```python
from build123d import *

# Parameters (mm, degrees)
F0_R         = 3.5
F0_R_2       = 2.8
F1_DEPTH     = 12
F3_DEPTH     = 1.7
F5_DEPTH     = 0.7
F6_T4_DEPTH  = 6.526963201
F6_S5_R      = 2.8
F6_T6_DEPTH  = 5
F6_T10_DEPTH = 6.526963201
F6_S11_R     = 2.8
F6_T12_DEPTH = 5
F6_T16_DEPTH = 6.526963201
F6_S17_R     = 2.8
F6_T18_DEPTH = 5
F6_T22_DEPTH = 6.526963201
F6_S23_R     = 2.8
F6_T24_DEPTH = 5
F7_T2_ANGLE  = 236.1398810925
F7_T4_ANGLE  = 236.1398810925


# Not quite as in the source:
# - a fillet or chamfer that OpenCascade refuses, or shapes differently, is made with other operations: its cross-section is extruded or revolved along the edge and cut away or added
# - a pattern or mirror of a feature is missing from the dataset's text; its kind, count and spacing are read off the source's solid


with BuildPart() as f1:
    # F0 (on Top) → F1 (new body)
    with BuildSketch(Plane.XY):
        Polygon((3.1971086236, -5.9505038819), (6.7518418389, -0.2064746542), (3.5547332152, 5.7440292277), (-3.1971086236, 5.9505038819), (-6.7518418389, 0.2064746542), (-3.5547332152, -5.7440292277), align=None)
        Circle(F0_R, mode=Mode.SUBTRACT)
        Circle(F0_R)
        Circle(F0_R_2, mode=Mode.SUBTRACT)
    extrude(amount=F1_DEPTH)

    # F2 (on face) → F3 (cut)
    with BuildSketch(Plane(origin=(0, 0, 0), x_dir=(1, 0, 0), z_dir=(0, 0, -1))):
        with BuildLine():
            Line((-5.3518418389, -1.1), (-2.5748786379, -1.1))
            ThreePointArc((-2.5748786379, -1.1), (-2.8, 0), (-2.5748786379, 1.1))
            Line((-2.5748786379, 1.1), (-5.3518418389, 1.1))
            Line((-5.3518418389, 1.1), (-5.3518418389, -1.1))
        make_face()
        with BuildLine():
            Line((2.5748786379, -1.1), (5.3518418389, -1.1))
            Line((5.3518418389, -1.1), (5.3518418389, 1.1))
            Line((5.3518418389, 1.1), (2.5748786379, 1.1))
            ThreePointArc((2.5748786379, 1.1), (2.7431423756, 0.5613999527), (2.8, 0))
            ThreePointArc((2.8, 0), (2.7431423756, -0.5613999527), (2.5748786379, -1.1))
        make_face()
    extrude(amount=-F3_DEPTH, mode=Mode.SUBTRACT)

    # F4 (on face) → F5 (join)
    with BuildSketch(Plane(origin=(0, 0, 0), x_dir=(1, 0, 0), z_dir=(0, 0, -1))):
        with BuildLine():
            ThreePointArc((-3.6402666737, -1.1), (0, -3.8028333457), (3.6402666737, -1.1))
            Line((3.6402666737, -1.1), (2.5748786379, -1.1))
            ThreePointArc((2.5748786379, -1.1), (0, -2.8), (-2.5748786379, -1.1))
            Line((-2.5748786379, -1.1), (-3.6402666737, -1.1))
        make_face()
    f5 = extrude(amount=F5_DEPTH)

    # F5_copies: F5 across plane
    add(f5.mirror(Plane(origin=(0, 0, 0), x_dir=(0, 0, -1), z_dir=(0, -1, 0))))

    # F6: fillet of radius 1.5 on 4 edges, made by hand


with BuildPart() as f6_tool2:
    # F6_s3 → F6_t4 (new body)
    with BuildSketch(Plane.YZ.offset(-1.1751213621)):
        with BuildLine():
            ThreePointArc((1.1, 0.2), (0.6606601718, 1.2606601718), (-0.4, 1.7))
            Line((-0.4, 1.7), (1.1, 1.7))
            Line((1.1, 1.7), (1.1, 0.2))
        make_face()
    extrude(amount=F6_T4_DEPTH)

    # F6_s5 → F6_t6 (cut, symmetric)
    with BuildSketch(Plane.XY.offset(1)):
        Circle(F6_S5_R)
    extrude(amount=F6_T6_DEPTH, both=True, mode=Mode.SUBTRACT)


with BuildPart() as f1_1:
    add(f1.part)

    # F6_t1: union F6_tool2
    add(f6_tool2.part)


with BuildPart() as f6_tool8:
    # F6_s9 → F6_t10 (new body)
    with BuildSketch(Plane.YZ.offset(-5.3518418389)):
        with BuildLine():
            ThreePointArc((1.1, 0.2), (0.6606601718, 1.2606601718), (-0.4, 1.7))
            Line((-0.4, 1.7), (1.1, 1.7))
            Line((1.1, 1.7), (1.1, 0.2))
        make_face()
    extrude(amount=F6_T10_DEPTH)

    # F6_s11 → F6_t12 (cut, symmetric)
    with BuildSketch(Plane.XY.offset(1)):
        Circle(F6_S11_R)
    extrude(amount=F6_T12_DEPTH, both=True, mode=Mode.SUBTRACT)


with BuildPart() as f1_2:
    add(f1_1.part)

    # F6_t7: union F6_tool8
    add(f6_tool8.part)


with BuildPart() as f6_tool14:
    # F6_s15 → F6_t16 (new body)
    with BuildSketch(Plane.YZ.offset(5.3518418389)):
        with BuildLine():
            ThreePointArc((-1.1, 0.2), (-0.6606601718, 1.2606601718), (0.4, 1.7))
            Line((0.4, 1.7), (-1.1, 1.7))
            Line((-1.1, 1.7), (-1.1, 0.2))
        make_face()
    extrude(amount=-F6_T16_DEPTH)

    # F6_s17 → F6_t18 (cut, symmetric)
    with BuildSketch(Plane.XY.offset(1)):
        Circle(F6_S17_R)
    extrude(amount=F6_T18_DEPTH, both=True, mode=Mode.SUBTRACT)


with BuildPart() as f1_3:
    add(f1_2.part)

    # F6_t13: union F6_tool14
    add(f6_tool14.part)


with BuildPart() as f6_tool20:
    # F6_s21 → F6_t22 (new body)
    with BuildSketch(Plane.YZ.offset(1.1751213621)):
        with BuildLine():
            ThreePointArc((-1.1, 0.2), (-0.6606601718, 1.2606601718), (0.4, 1.7))
            Line((0.4, 1.7), (-1.1, 1.7))
            Line((-1.1, 1.7), (-1.1, 0.2))
        make_face()
    extrude(amount=-F6_T22_DEPTH)

    # F6_s23 → F6_t24 (cut, symmetric)
    with BuildSketch(Plane.XY.offset(1)):
        Circle(F6_S23_R)
    extrude(amount=F6_T24_DEPTH, both=True, mode=Mode.SUBTRACT)


with BuildPart() as f1_4:
    add(f1_3.part)

    # F6_t19: union F6_tool20
    add(f6_tool20.part)

    # F7: fillet of radius 1 on 2 edges, made by hand

    # F7_s1 → F7_t2 (revolve, cut)
    with BuildSketch(Plane(origin=(0, 0, 0), x_dir=(0, 0, 1), z_dir=(-0.4705490205, -0.8823738546, 0))):
        with BuildLine():
            ThreePointArc((0.3, -2.8), (-0.4071067812, -3.0928932188), (-0.7, -3.8))
            Line((-0.7, -3.8), (-0.7, -2.8))
            Line((-0.7, -2.8), (0.3, -2.8))
        make_face()
    revolve(axis=Axis((0, 0, -0.7), (0, 0, 1)), revolution_arc=F7_T2_ANGLE, mode=Mode.SUBTRACT)

    # F7_s3 → F7_t4 (revolve, cut)
    with BuildSketch(Plane(origin=(0, 0, 0), x_dir=(0, 0, 1), z_dir=(-0.4705490205, 0.8823738546, 0))):
        with BuildLine():
            ThreePointArc((0.3, 2.8), (-0.4071067812, 3.0928932188), (-0.7, 3.8))
            Line((-0.7, 3.8), (-0.7, 2.8))
            Line((-0.7, 2.8), (0.3, 2.8))
        make_face()
    revolve(axis=Axis((0, 0, -0.7), (0, 0, -1)), revolution_arc=F7_T4_ANGLE, mode=Mode.SUBTRACT)


solid = f1_4.part
```
Could you check a few things on this model? Use its own coordinates, in mm. A direction names the side the tool comes from. Coordinates: 2 decimals unless noted, no trailing zeros. Write each loop counter-clockwise with the first axis right and the second up, starting at its lowest first coordinate (ties: lowest second). Pieces come first, ordered by that corner, then holes. Notation, with made-up numbers: M -24,55.5 L -4,55.5 A20 ccw -4,68.5 Z; hole C 16,-20 d10. An arc over 180 degrees is marked long. Answer as CSV lines item,"result". Start each with the question number.
1) Please list where these lines run through material, in increasing order: line 1 (Z direction, x = 3, y = 3.25); line 2 (Y direction, x = 2.5, z = 9.25); line 3 (Y direction, x = 0, z = 7). Write a range as from..to.
2) We'd pull the mould along X, two halves only. Please class faces 1 (the flat face through (3, -1.1, 0)), 2 (the flat face through (3, 0, 12)), 3 (the flat face through (-4.95, 3.12, 5.92)): +X half, -X half, draft (parallel to the pull), parting line (faces both ways), or undercut.
3) I want a section at D-D, the plane z = 1. Please give me the cut outline in (x, y), and give its area (3 significant figures).
4) For faces 4 (the cylindrical face through (-0.1, -3.8, -0.3)), 5 (the flat face through (5.176, 2.727, 5.916)), 6 (the flat face through (-5.176, -2.727, 5.916)), 7 (the cylindrical face through (-0.1, 3.8, -0.3)), 8 (the cylindrical face through (4, -0.8, 1.1)), which set-ups out of +Z, -Z, +X, -X, +Y, -Y let a thin tool reach every point of the face, with its end or its side?
5) I want a section at A-A, the plane z = 11. Please give me the cut outline in (x, y), and give its area (3 significant figures).
6) For P1, Ø0.5, axis at x = -4, z = 0, coming from the -Y side; P2, Ø2, axis at y = -4, z = 9.5, coming from the -X side; P3, Ø0.8, axis at y = -0.5, z = 1, coming from the -X side; P4, Ø5, axis at x = 4, z = 5, coming from the -Y side, each with a flat end and sliding along its axis, tell me the tip position at first contact or that it passes through.
7) I want a section at C-C, the plane x = -4.25. Please give me the cut outline in (y, z), and give its area (3 significant figures).
Data:
1,line 1,"z = 0..12"
1,line 2,"y = -5.93..-1.26, 1.26..5.78"
1,line 3,"y = -5.85..-2.8, 2.8..5.85"
2,face 1,"undercut"
2,face 2,"draft"
2,face 3,"-X half"
3,outline,"M -6.75,0.21 L -3.55,-5.74 L 3.2,-5.95 L 6.75,-0.21 L 3.55,5.74 L -3.2,5.95 Z; hole M -5.35,-0.87 L -2.66,-0.87 A2.8 ccw 2.66,-0.87 L 5.35,-0.87 L 5.35,0.87 L 2.66,0.87 A2.8 ccw -2.66,0.87 L -5.35,0.87 Z"
3,area,"84.9 mm^2"
4,face 4,"-Z, -Y"
4,face 5,"+Z, -Z, +X, +Y"
4,face 6,"+Z, -Z, -X, -Y"
4,face 7,"-Z, +Y"
4,face 8,"-Z"
5,outline,"M -6.75,0.21 L -3.55,-5.74 L 3.2,-5.95 L 6.75,-0.21 L 3.55,5.74 L -3.2,5.95 Z; hole C 0,0 d5.6"
5,area,"93.9 mm^2"
6,P1,"stops at y = -5.38"
6,P2,"stops at x = -5.03"
6,P3,"stops at x = -6.59"
6,P4,"stops at y = -5.95"
7,outline,"M -4.45,0 L -1.1,0 L -1.1,0.2 A1.5 cw 0,1.65 A1.5 cw 1.1,0.2 L 1.1,0 L 4.25,0 L 4.25,12 L -4.45,12 Z"
7,area,"102 mm^2"
